Here's how the part is built. I have some questions about the finished solid (model axes, mm). A direction names the side the tool comes from. Round coordinates to 2 decimals unless told otherwise and drop trailing zeros. Order: outer loops, then holes, each group sorted by start corner. A loop starts at its lowest first (then second) coordinate and runs counter-clockwise, first axis right, second up. Notation, with made-up numbers: (18, -12.75) -> (37, -12.75) arc R13 cw to (37, 6.25) -> close; hole circle Ø10 at (-6.5, 74.5). An arc over 180 degrees is marked (long way). Use a Markdown table: item, result. Add a question column.
(1) Thinking about a two-plate mould opening in Z: for faces 4 (the face through (-0.74, 3.35, 9.39)), 5 (the face through (-3, 7, 0)), 6 (the face through (-2.26, 5.89, 16.09)), which applies, pulls with the +Z half, pulls with the -Z half, needs draft (parallel to the pull), parting line crosses it, or undercut?
(2) I'm going to push flat-ended pins straight in: P1, Ø4, axis at x = -13.5, z = 12.5, coming from the -Y side; P2, Ø1.5, axis at x = -11.5, z = 6, coming from the +Y side; P3, Ø2, axis at y = -1, z = 12.5, coming from the +X side; P4, Ø4, axis at x = -2.5, z = 13, coming from the +Y side. Where does each tip first touch, or does it pass through?
(3) If I drill on probe 1 along Z at (x, y) = (-13, 3.25); probe 2 along X at (y, z) = (2, 14.5); probe 3 along Y at (x, z) = (0, 12), over which ranges is the centre line in solid material (lowest first)?
(4) I want a section at B-B, the plane y = -0.5. Please give me the cut outline in (x, z), then the cut area to 3 significant figures.
(5) I want a section at C-C, the plane x = 2.25. Give the number of separate pieces and of enclosed holes in the cut face, then the cut area to 3 significant figures.
(6) On a 3-axis mill with a long thin cutter (end or side, diameter ignored), from which of +Z, -Z, +X, -X, +Y, -Y can I reach the whole of each face in a straight line? I mean faces 1 (the face through (5.26, 12.2, 3.39)), 2 (the face through (-13, 0.794, 9)), 3 (the face through (-16.33, 1.86, 9.66)). Say none if no direction works.
Autodesk Inventor part; units mm, degrees
ref_plane "YZ Plane" through (0, 0, 0) normal (1, 0, 0) x (0, 1, 0)
ref_plane "XZ Plane" through (0, 0, 0) normal (0, 1, 0) x (-1, 0, 0)
ref_plane "XY Plane" through (0, 0, 0) normal (0, 0, 1) x (1, 0, 0)
sketch "Sketch3" plane through (0, 0, 0) normal (0, 0, 1) x (1, 0, 0)
  circle A0 centre (0, 0) radius 3.429
  circle A1 centre (0, 0) radius 6.35
  line L0 (6.35, 22.225) -> (-19.1908, 0.7937)
  line L1 (-19.1908, 0.7937) -> (-6.3002, 0.7937)
  line L2 (6.35, 22.225) -> (6.35, 0)
  dimension "d23" = 6.858
  dimension "d24" = 12.7
  dimension "d27" = 0.7937
  dimension "d28" = 6.35
  dimension "d29" = 50
  dimension "d30" = 22.225
extrude "Extrusion3" add sketch "Sketch3" along normal blind 19.05
fillet "Fillet2" radius 6.35 1 edges at (-6.3002, 0.7938, 9.525)
sketch "Sketch4" plane through (-19.1908, 0.7938, 19.05) normal (-0.6427876, 0.7660444, 0) x (0.7660444, 0.6427876, 0)
  line L0 (33.3411, 0) -> (0, 0)
  line L1 (6.35, 0) -> (6.35, 18.8766) construction
  line L2 (0, 19.05) -> (0, 0)
  line L3 (0, 9.525) -> (33.3411, 9.525) construction
  line L4 (33.3411, 19.05) -> (33.3411, 0)
  point P0 (14.1908, 19.05)
  point P1 (6.35, 3.175)
  point P2 (6.35, 15.875)
  point P3 (16.1742, 15.875)
  point P4 (16.1742, 3.175)
  point P5 (25.9983, 15.875)
  point P6 (25.9983, 3.175)
  dimension "d33" = 6.35
  dimension "d34" = 3.175
  dimension "d45" = 9.8242
hole "Hole1" at (-14.3264, 4.8755, 15.875) at (-14.3264, 4.8755, 3.175) at (-6.8006, 11.1903, 15.875) at (-6.8006, 11.1903, 3.175) at (0.7251, 17.5052, 3.175) at (0.7251, 17.5052, 15.875) direction (0.6427876, -0.7660444, 0) diameter 2.54 depth 6.35 tip angle 118
fillet "Fillet4" radius 1.5875 2 edges at (-19.1908, 0.7937, 9.525) (6.35, 22.225, 9.525)
properties part number "Wedge Mount" material "UHMW, White"
Taken from the geometry:
| question | item | result |
|---|---|---|
| 1 | face 4 | needs draft |
| 1 | face 5 | pulls with the -Z half |
| 1 | face 6 | undercut |
| 2 | P1 | stops at y = 0.79 |
| 2 | P2 | stops at y = 7.88 |
| 2 | P3 | stops at x = 6.35 |
| 2 | P4 | stops at y = 16.48 |
| 3 | probe 1 | z = 0 to 1.91, 4.44 to 14.61, 17.14 to 19.05 |
| 3 | probe 2 | x = -16.37 to -2.79, 2.79 to 6.35 |
| 3 | probe 3 | y = -6.35 to -3.43, 3.43 to 16.9 |
| 4 | outline | (-7.58, 0) -> (-3.39, 0) -> (-3.39, 19.05) -> (-7.58, 19.05) -> close; (3.39, 0) -> (6.33, 0) -> (6.33, 19.05) -> (3.39, 19.05) -> close |
| 4 | area | 136 mm2 |
| 5 | separate pieces | 2 |
| 5 | enclosed holes | 2 |
| 5 | area | 357 mm2 |
| 6 | face 1 | none |
| 6 | face 2 | +Z, -Z, -X, -Y |
| 6 | face 3 | +Z, -Z, -X |
